Geometry check sheet. Reference: the model listing, model coordinates, mm. Give positions to 0.01 mm unless a question says otherwise; leave off trailing zeros. One line per question, with ' | ' between items. Start each with the question number.
from build123d import *

# Parameters (mm, degrees)
F1_DEPTH = 4


# Not quite as in the source:
# - ends of sketch curves that miss each other by under 0.0002 mm in the source are joined


with BuildPart() as f1:
    # F0 (on Front) → F1 (new body)
    with BuildSketch(Plane.XZ):
        Polygon((48.878435, 1.5), (-48.878435, 1.5), (-48.878435, -1.5), (-46.5690339232, -1.5), (-46.4310674122, -1.5), (-44.1216663354, -1.5), (-43.9836963354, -1.5), (-41.6742952587, -1.5), (-41.5363252587, -1.5), (-39.22692239, -1.5), (-39.08895239, -1.5), (-36.7795513132, -1.5), (-36.6415813132, -1.5), (-34.3321802365, -1.5), (-34.1942102365, -1.5), (-31.8848091597, -1.5), (-31.7468391597, -1.5), (-29.4374380829, -1.5), (-29.2994680829, -1.5), (-26.9900670062, -1.5), (-26.8520970062, -1.5), (-24.5426959294, -1.5), (-24.4047259294, -1.5), (-22.0953248527, -1.5), (-21.9573548527, -1.5), (-19.6479537759, -1.5), (-19.5099837759, -1.5), (-17.2005822649, -1.5), (-17.062612265, -1.5), (-14.7532111882, -1.5), (-14.6152411882, -1.5), (-12.3058401114, -1.5), (-12.1678701114, -1.5), (-9.8584690347, -1.5), (-9.7204990347, -1.5), (-7.4110979579, -1.5), (-7.2731279579, -1.5), (-4.9637268812, -1.5), (-4.8257568812, -1.5), (-2.5163558044, -1.5), (-2.3783858044, -1.5), (-0.0689847276, -1.5), (0.0689852724, -1.5), (2.3783863491, -1.5), (2.5163563491, -1.5), (4.8257574259, -1.5), (4.9637274259, -1.5), (7.2731285026, -1.5), (7.4110985026, -1.5), (9.7204995794, -1.5), (9.8584695794, -1.5), (12.1678706561, -1.5), (12.3058406561, -1.5), (14.6152417329, -1.5), (14.7532117329, -1.5), (17.0626128097, -1.5), (17.2005828097, -1.5), (19.5099838864, -1.5), (19.6479538864, -1.5), (21.5619457761, -1.5), (21.9573549632, -1.5), (22.0953249632, -1.5), (23.8713468528, -1.5), (24.4047260399, -1.5), (24.5426960399, -1.5), (26.8520971167, -1.5), (26.9900671167, -1.5), (29.2994681935, -1.5), (29.4374381935, -1.5), (31.7468392702, -1.5), (31.8848092702, -1.5), (34.194210347, -1.5), (34.332180347, -1.5), (36.6415814237, -1.5), (36.7795514237, -1.5), (39.0889525005, -1.5), (39.2269225005, -1.5), (41.5363235773, -1.5), (41.6742935773, -1.5), (43.983694654, -1.5), (44.121664654, -1.5), (46.4310657308, -1.5), (46.5690357308, -1.5), (48.878435, -1.5), align=None)
        Polygon((-46.5690339232, -1.5), (-48.878435, -1.5), (-47.7237344616, -3.5), align=None)
        Polygon((47.7237362691, -3.5), (48.8784368075, -1.5), (46.5690357308, -1.5), align=None)
        Polygon((-44.1216663354, -1.5), (-46.4310674122, -1.5), (-45.2763668738, -3.5), align=None)
        Polygon((45.2763651924, -3.5), (46.4310657308, -1.5), (44.121664654, -1.5), align=None)
        Polygon((-41.6742952587, -1.5), (-43.9836963354, -1.5), (-42.8289957971, -3.5), align=None)
        Polygon((42.8289941156, -3.5), (43.983694654, -1.5), (41.6742935773, -1.5), align=None)
        Polygon((-39.22692239, -1.5), (-41.5363252587, -1.5), (-40.3816238243, -3.5), align=None)
        Polygon((40.3816230389, -3.5), (41.5363235773, -1.5), (39.2269225005, -1.5), align=None)
        Polygon((-36.7795513132, -1.5), (-39.08895239, -1.5), (-37.9342518516, -3.5), align=None)
        Polygon((37.9342519621, -3.5), (39.0889525005, -1.5), (36.7795514237, -1.5), align=None)
        Polygon((-34.3321802365, -1.5), (-36.6415813132, -1.5), (-35.4868807748, -3.5), align=None)
        Polygon((35.4868808854, -3.5), (36.6415814237, -1.5), (34.332180347, -1.5), align=None)
        Polygon((-31.8848091597, -1.5), (-34.1942102365, -1.5), (-33.0395096981, -3.5), align=None)
        Polygon((33.0395098086, -3.5), (34.194210347, -1.5), (31.8848092702, -1.5), align=None)
        Polygon((-29.4374380829, -1.5), (-31.7468391597, -1.5), (-30.5921386213, -3.5), align=None)
        Polygon((30.5921387318, -3.5), (31.7468392702, -1.5), (29.4374381935, -1.5), align=None)
        Polygon((-26.9900670062, -1.5), (-29.2994680829, -1.5), (-28.1447675446, -3.5), align=None)
        Polygon((28.1447676551, -3.5), (29.2994681935, -1.5), (26.9900671167, -1.5), align=None)
        Polygon((-24.5426959294, -1.5), (-26.8520970062, -1.5), (-25.6973964678, -3.5), align=None)
        Polygon((25.6973965783, -3.5), (26.8520971167, -1.5), (24.5426960399, -1.5), align=None)
        Polygon((-22.0953248527, -1.5), (-24.4047259294, -1.5), (-23.250025391, -3.5), align=None)
        Polygon((23.2500255016, -3.5), (24.4047260399, -1.5), (23.8713468528, -1.5), (22.0953249632, -1.5), align=None)
        Polygon((-19.6479537759, -1.5), (-21.9573548527, -1.5), (-20.8026543143, -3.5), align=None)
        Polygon((20.8026544248, -3.5), (21.9573549632, -1.5), (21.5619457761, -1.5), (19.6479538864, -1.5), align=None)
        Polygon((-17.2005822649, -1.5), (-19.5099837759, -1.5), (-18.3552830204, -3.500000376), align=None)
        Polygon((-14.7532111882, -1.5), (-17.062612265, -1.5), (-15.9079117266, -3.5), align=None)
        Polygon((18.355283348, -3.5), (19.5099838864, -1.5), (17.2005828097, -1.5), align=None)
        Polygon((-12.3058401114, -1.5), (-14.6152411882, -1.5), (-13.4605406498, -3.5), align=None)
        Polygon((15.9079122713, -3.5), (17.0626128097, -1.5), (14.7532117329, -1.5), align=None)
        Polygon((-9.8584690347, -1.5), (-12.1678701114, -1.5), (-11.0131695731, -3.5), align=None)
        Polygon((13.4605411945, -3.5), (14.6152417329, -1.5), (12.3058406561, -1.5), align=None)
        Polygon((-7.4110979579, -1.5), (-9.7204990347, -1.5), (-8.5657984963, -3.5), align=None)
        Polygon((11.0131701178, -3.5), (12.1678706561, -1.5), (9.8584695794, -1.5), align=None)
        Polygon((-4.9637268812, -1.5), (-7.2731279579, -1.5), (-6.1184274195, -3.5), align=None)
        Polygon((8.565799041, -3.5), (9.7204995794, -1.5), (7.4110985026, -1.5), align=None)
        Polygon((-2.5163558044, -1.5), (-4.8257568812, -1.5), (-3.6710563428, -3.5), align=None)
        Polygon((6.1184279642, -3.5), (7.2731285026, -1.5), (4.9637274259, -1.5), align=None)
        Polygon((-0.0689847276, -1.5), (-2.3783858044, -1.5), (-1.223685266, -3.5), align=None)
        Polygon((3.6710568875, -3.5), (4.8257574259, -1.5), (2.5163563491, -1.5), align=None)
        Polygon((2.3783863491, -1.5), (0.0689852724, -1.5), (1.2236858107, -3.5), align=None)
    extrude(amount=F1_DEPTH)


solid = f1.part
Item 1: Depth check by flat-ended pin: pin 1 (1 mm diameter, centred on x = -37.5, y = -2, fed in from -Z); pin 2 (1 mm diameter, centred on x = -12.5, y = -2.5, fed in from -Z). Enter the tip coordinate at first touch or a pass-through.
Item 2: Cross-section at A-A, the plane z = -2.7. State how many separate pieces and enclosed holes the cut face has, plus the area to 3 significant figures.
Item 3: Material ranges on line 1 along Z through (x, y) = (24.5, -3.65); line 2 along Z through (x, y) = (26.5, -2.1), recorded low to high.
Outcome:
1) pin 1: stops at z = -3.5 | pin 2: stops at z = -2.7
2) separate pieces: 40 | enclosed holes: 0 | area: 148 mm²
3) line 1: z = -1.5 to 1.5 | line 2: z = -2.11 to 1.5
